For this review, take the finished solid that the model builds, in its own axes (mm). Give positions to 0.01 mm unless a question says otherwise; leave off trailing zeros. Write each loop counter-clockwise with the first axis right and the second up, starting at its lowest first coordinate (ties: lowest second). Pieces come first, ordered by that corner, then holes.
1) For P1, Ø4.5, axis at x = 78.5, y = 46.5, coming from the -Z side; P2, Ø1, axis at x = 24.5, z = -11.5, coming from the +Y side; P3, Ø1, axis at x = 3.5, y = 24, coming from the -Z side; P4, Ø8, axis at y = -17.5, z = -12, coming from the +X side (3 decimals), all flat-tipped, find the tip position at first contact; note any pin that passes through.
2) We need section B-B on y = 15.78. Give the boundary of the cut face in (x, z) (3 decimals), and give its area (3 significant figures).
3) We need section D-D on y = -45.92. Give the boundary of the cut face in (x, z) (3 decimals).
4) Wall thickness on line 1 along Z through (x, y) = (-22, 20): over which ranges is the line inside the solid? List them lowest first.
5) We need section A-A on z = -10.75. Give the boundary of the cut face in (x, y) (3 decimals).
6) We need section C-C on x = -37. Give the boundary of the cut face in (y, z).
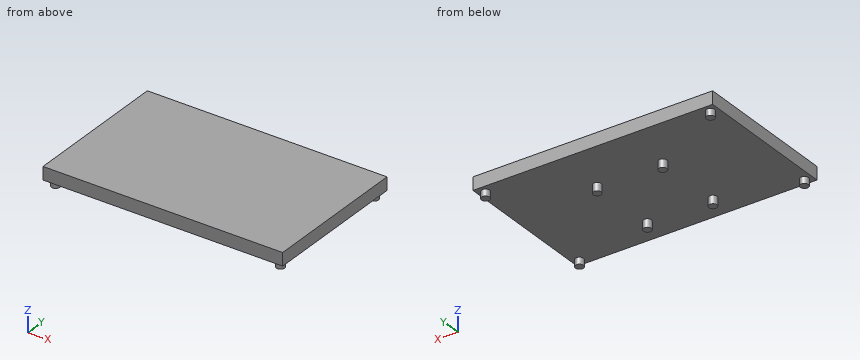
from build123d import *

# Parameters (mm, degrees)
SKETCH1_W           = 164.89
SKETCH1_H           = 102
BOSS_EXTRUDE1_DEPTH = 8.89
SKETCH2_R           = 2.794
BOSS_EXTRUDE2_DEPTH = 4.572
SKETCH3_R           = 2.794
BOSS_EXTRUDE3_DEPTH = 5.588


with BuildPart() as part:
    # Sketch1 → Boss-Extrude1 (new body)
    with BuildSketch(Plane.XY):
        Rectangle(SKETCH1_W, SKETCH1_H)
    extrude(amount=-BOSS_EXTRUDE1_DEPTH)

    # Sketch2 → Boss-Extrude2 (add)
    with BuildSketch(Plane(origin=(0, 0, -8.89), x_dir=(-1, 0, 0), z_dir=(0, 0, -1))):
        with Locations(Location((-77.365, 45.92, 0), (0, 0, 180))):
            Circle(SKETCH2_R)
        with Locations(Location((77.365, 45.92, 0), (0, 0, 180))):
            Circle(SKETCH2_R)
        with Locations(Location((-77.365, -45.92, 0), (0, 0, 180))):
            Circle(SKETCH2_R)
        with Locations(Location((77.365, -45.92, 0), (0, 0, 180))):
            Circle(SKETCH2_R)
    extrude(amount=BOSS_EXTRUDE2_DEPTH)

    # Sketch3 → Boss-Extrude3 (add)
    with BuildSketch(Plane(origin=(0, 0, -8.89), x_dir=(-1, 0, 0), z_dir=(0, 0, -1))):
        with Locations(Location((-21.739, 15.78, 0), (0, 0, 180))):
            Circle(SKETCH3_R)
        with Locations(Location((-21.739, -33.22, 0), (0, 0, 180))):
            Circle(SKETCH3_R)
        with Locations(Location((23.351, -33.22, 0), (0, 0, 180))):
            Circle(SKETCH3_R)
        with Locations(Location((23.351, 15.78, 0), (0, 0, 180))):
            Circle(SKETCH3_R)
    extrude(amount=BOSS_EXTRUDE3_DEPTH)


solid = part.part
Results list:
1. P1: stops at z = -13.46
1. P2: stops at y = 17.42
1. P3: stops at z = -8.89
1. P4: stops at x = 82.445
2. outline: (-82.445, -8.89) - (-26.145, -8.89) - (-26.145, -14.478) - (-20.557, -14.478) - (-20.557, -8.89) - (18.945, -8.89) - (18.945, -14.478) - (24.533, -14.478) - (24.533, -8.89) - (82.445, -8.89) - (82.445, 0) - (-82.445, 0) - close
2. area: 1,530 mm2
3. outline: (-82.445, -8.89) - (-80.159, -8.89) - (-80.159, -13.462) - (-74.571, -13.462) - (-74.571, -8.89) - (74.571, -8.89) - (74.571, -13.462) - (80.159, -13.462) - (80.159, -8.89) - (82.445, -8.89) - (82.445, 0) - (-82.445, 0) - close
4. line 1: z = -8.89 to 0
5. outline: circle Ø5.588 at (-77.365, -45.92); circle Ø5.588 at (-77.365, 45.92); circle Ø5.588 at (-23.351, -33.22); circle Ø5.588 at (-23.351, 15.78); circle Ø5.588 at (21.739, -33.22); circle Ø5.588 at (21.739, 15.78); circle Ø5.588 at (77.365, -45.92); circle Ø5.588 at (77.365, 45.92)
6. outline: (-51, -8.89) - (51, -8.89) - (51, 0) - (-51, 0) - close
